Could you check a few things on this model? Use its own coordinates, in mm. A direction names the side the tool comes from. Give positions to 0.01 mm unless a question says otherwise; leave off trailing zeros. Write each loop counter-clockwise with the first axis right and the second up, starting at its lowest first coordinate (ties: lowest second). Pieces come first, ordered by that corner, then holes. Notation, with made-up numbers: (43.25, -27) - (99.25, -27) arc R31 ccw to (99.25, -3) - close; hole circle Ø6 at (61, -33). An arc over 180 degrees is marked (long way). Answer as a JSON object with one key per item and string values. Group by question number.
```python
from build123d import *

# Parameters (mm, degrees)
SKETCH_W        = 80
SKETCH_H        = 76
SKETCH_W_2      = 32
SKETCH_H_2      = 53.5
PAD_DEPTH       = 7
SKETCH001_W     = 80
SKETCH001_H     = 76
SKETCH001_W_2   = 65
SKETCH001_H_2   = 66
PAD001_DEPTH    = 35
PAD005_DEPTH    = 5
SKETCH008_W     = 50.2
SKETCH008_H     = 5.3
POCKET_DEPTH    = 5
SKETCH012_R     = 3.1
POCKET003_DEPTH = 10
SKETCH013_W     = 35
SKETCH013_H     = 56
SKETCH013_W_2   = 30
SKETCH013_H_2   = 52
PAD008_DEPTH    = 3


with BuildPart() as part:
    # Sketch → Pad (new body)
    with BuildSketch(Plane.XZ):
        with Locations((0, 38)):
            Rectangle(SKETCH_W, SKETCH_H)
        with Locations((-0.1, 38)):
            Rectangle(SKETCH_W_2, SKETCH_H_2, mode=Mode.SUBTRACT)
    extrude(amount=PAD_DEPTH)

    # Sketch001 (on Face9 of Pad) → Pad001 (join)
    with BuildSketch(Plane(origin=(0, 0, 0), x_dir=(1, 0, 0), z_dir=(0, 1, 0))):
        with Locations((0, -38)):
            Rectangle(SKETCH001_W, SKETCH001_H)
        with Locations((2.5, -38)):
            Rectangle(SKETCH001_W_2, SKETCH001_H_2, mode=Mode.SUBTRACT)
    extrude(amount=PAD001_DEPTH)

    # Sketch005 (on Face12 of Pad001) → Pad005 (join)
    with BuildSketch(Plane(origin=(0, 0, 0), x_dir=(1, 0, 0), z_dir=(0, 0, -1))):
        Polygon((-40, -35), (-40, 7), (-35, -6.75), (-35, -35), align=None)
    extrude(amount=PAD005_DEPTH)

    # Sketch008 (on Face18 of Pad005) → Pocket (cut)
    with BuildSketch(Plane(origin=(-40, 0, 0), x_dir=(0, 0, -1), z_dir=(-1, 0, 0))):
        with Locations((-20.1, -15.5)):
            Rectangle(SKETCH008_W, SKETCH008_H)
    extrude(amount=-POCKET_DEPTH, mode=Mode.SUBTRACT)

    # Sketch012 (on Face16 of Pocket) → Pocket003 (cut)
    with BuildSketch(Plane(origin=(-40, 0, 0), x_dir=(0, 0, -1), z_dir=(-1, 0, 0))):
        with Locations((-30, -26)):
            Circle(SKETCH012_R)
    extrude(amount=-POCKET003_DEPTH, mode=Mode.SUBTRACT)

    # Sketch013 (on Face3 of Pocket003) → Pad008 (join)
    with BuildSketch(Plane(origin=(0, 0, 0), x_dir=(1, 0, 0), z_dir=(0, 1, 0))):
        with Locations((0, -38)):
            Rectangle(SKETCH013_W, SKETCH013_H)
        with Locations((0, -38)):
            Rectangle(SKETCH013_W_2, SKETCH013_H_2, mode=Mode.SUBTRACT)
    extrude(amount=PAD008_DEPTH)


with BuildPart() as part_1:
    # Body placement: moved
    add(part.part.moved(Location((0, -43, 0))))


solid = part_1.part
```
(1) If we mould it in two halves opening along Z, with no side actions, what happens to faces 1 (the flat face through (-20, -43, 38)), 2 (the flat face through (2, -26, 71)), 3 (the flat face through (-38, -38, -5)), 4 (the flat face through (36, -8, 36))? For each: +Z half, -Z half, draft (parallel to the pull), parting line (faces both ways), or undercut.
(2) I need wall thicknesses on L1, parallel to Z at x = 10.5, y = -42; L2, parallel to X at y = -42, z = 55; L3, parallel to X at y = -10.5, z = 45. Which ranges of each line are inside material? Lowest first, please.
(3) I want a section at B-B, the plane y = -28.5. Please give me the cut outline in (x, z), and give its area (3 significant figures).
(4) For faces 5 (the flat face through (-35, -33, -2)), 6 (the flat face through (-15.6, -43, 37.9)), 7 (the cylindrical face through (-35.1, -17.1, 33.1)), 8 (the flat face through (17.5, -42, 38)), 9 (the flat face through (-38, -24.85, 20)), which set-ups out of +Z, -Z, +X, -X, +Y, -Y let a thin tool reach every point of the face, with its end or its side?
(5) I want a section at D-D, the plane x = 19. Please give me the cut outline in (y, z).
(6) I want a section at A-A, the plane x = -1.5. Please give me the cut outline in (y, z), and give its area (4 significant figures).
(7) Will this pin go through, and if not, where does the flat tip stop? P1, Ø3, axis at x = 10.5, y = -22.5, coming from the -Z side.
(8) I want a section at C-C, the plane z = 32. Please give me the cut outline in (x, y).
Entries:
{
 "1": {"face 1": "undercut", "face 2": "undercut", "face 3": "-Z half", "face 4": "draft"},
 "2": {"L1": "0 to 5, 10 to 12, 64 to 66, 71 to 76", "L2": "-40 to -30, -17.5 to -15, 15 to 17.5, 35 to 40", "L3": "-40 to -30, 35 to 40"},
 "3": {"outline": "(-40, 45.2) - (-35, 45.2) - (-35, 0) - (40, 0) - (40, 76) - (-40, 76) - close; hole (-30, 5) - (35, 5) - (35, 71) - (-30, 71) - close", "area": "1,560 mm^2"},
 "4": {"face 5": "-Z, +X, +Y, -Y", "face 6": "-Y", "face 7": "-X", "face 8": "+Y", "face 9": "-Z, -X"},
 "5": {"outline": "(-50, 0) - (-8, 0) - (-8, 5) - (-43, 5) - (-43, 71) - (-8, 71) - (-8, 76) - (-50, 76) - close"},
 "6": {"outline": "(-50, 0) - (-8, 0) - (-8, 5) - (-43, 5) - (-43, 10) - (-40, 10) - (-40, 12) - (-43, 12) - (-43, 11.25) - (-50, 11.25) - close; (-50, 64.75) - (-43, 64.75) - (-43, 64) - (-40, 64) - (-40, 66) - (-43, 66) - (-43, 71) - (-8, 71) - (-8, 76) - (-50, 76) - close", "area": "519.5 mm^2"},
 "7": {"P1": "z = 0"},
 "8": {"outline": "(-40, -50) - (-16.1, -50) - (-16.1, -43) - (-15, -43) - (-15, -40) - (-17.5, -40) - (-17.5, -43) - (-30, -43) - (-30, -19.37) - (-40, -19.37) - (-40, -24.85) - (-35, -24.85) - (-35, -30.15) - (-40, -30.15) - close; (-40, -14.63) - (-30, -14.63) - (-30, -8) - (-40, -8) - close; (15, -43) - (15.9, -43) - (15.9, -50) - (40, -50) - (40, -8) - (35, -8) - (35, -43) - (17.5, -43) - (17.5, -40) - (15, -40) - close"}
}
